from build123d import *

# Parameters (mm, degrees)
SKETCH1_R           = 18
BOSS_EXTRUDE1_DEPTH = 70
SKETCH2_R           = 2.5
BOSS_EXTRUDE2_DEPTH = 16
SKETCH3_R           = 9.5
SKETCH3_R_2         = 2.5
BOSS_EXTRUDE3_DEPTH = 25
SKETCH4_R           = 9.5
SKETCH4_R_2         = 4
BOSS_EXTRUDE4_DEPTH = 10


with BuildPart() as part:
    # Sketch1 → Boss-Extrude1 (new body)
    with BuildSketch(Plane.XY):
        Circle(SKETCH1_R)
    extrude(amount=BOSS_EXTRUDE1_DEPTH)

    # Sketch2 → Boss-Extrude2 (add)
    with BuildSketch(Plane.XY.offset(70)):
        Circle(SKETCH2_R)
    extrude(amount=BOSS_EXTRUDE2_DEPTH)

    # Sketch3 → Boss-Extrude3 (add)
    with BuildSketch(Plane.XY.offset(70)):
        Circle(SKETCH3_R)
        Circle(SKETCH3_R_2, mode=Mode.SUBTRACT)
    extrude(amount=BOSS_EXTRUDE3_DEPTH)

    # Sketch4 → Boss-Extrude4 (add)
    with BuildSketch(Plane.XY.offset(95)):
        Circle(SKETCH4_R)
        Circle(SKETCH4_R_2, mode=Mode.SUBTRACT)
    extrude(amount=BOSS_EXTRUDE4_DEPTH)


solid = part.part
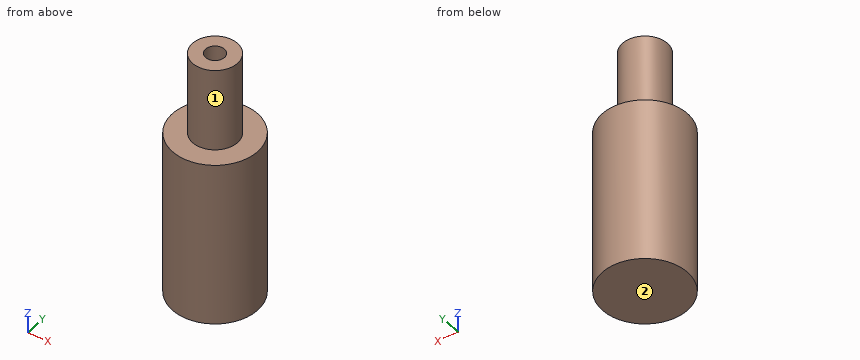
The listing builds one solid part. Answer for the finished solid, in the listing's coordinates (mm). Face numbers are marked on the shaded views. A direction names the side the tool comes from. Coordinates: 2 decimals unless noted, no trailing zeros. Order: outer loops, then holes, each group sorted by start corner. A loop starts at its lowest first (then second) coordinate and runs counter-clockwise, first axis right, second up.
Q1. Which of the six approach directions +Z, -Z, +X, -X, +Y, -Y give full straight-line access (tool end or side, diameter ignored) to the marked faces 1 and 2?
Q2. Given P1, Ø1, axis at y = -11, z = 27, coming from the -X side; P2, Ø2.5, axis at x = 1, y = 1, coming from the +Z side; P3, Ø1, axis at x = -10.5, y = -1.5, coming from the -Z side; P4, Ø6, axis at x = -13, z = 50, coming from the -Y side, each flat-ended and moving along its own axis, determine where each tip first touches the part or whether it passes through.
Q3. A cutting plane is placed at D-D, the plane z = 61. Write down the section's boundary in (x, y).
Q4. A cutting plane is placed at B-B, the plane z = 88.5. Write down the section's boundary in (x, y), and give its area (3 significant figures).
Q5. Consider line 1 (Y direction, x = 0, z = 89.5); line 2 (Y direction, x = 0, z = 101.5); line 3 (Z direction, x = 11, y = 11.5). Determine where each line is inside the solid, lowest interval first.
Q6. A cutting plane is placed at A-A, the plane x = 0. Write down the section's boundary in (y, z), and give its area (3 significant figures).
Answers follow:
1. face 1: +Z
1. face 2: -Z, +X, -X, +Y, -Y
2. P1: stops at x = -14.62
2. P2: stops at z = 95
2. P3: stops at z = 0
2. P4: stops at y = -14.97
3. outline: circle Ø36 at (0, 0)
4. outline: circle Ø19 at (0, 0); hole circle Ø5 at (0, 0)
4. area: 264 mm2
5. line 1: y = -9.5 to -2.5, 2.5 to 9.5
5. line 2: y = -9.5 to -4, 4 to 9.5
5. line 3: z = 0 to 70
6. outline: (-18, 0) - (18, 0) - (18, 70) - (9.5, 70) - (9.5, 105) - (4, 105) - (4, 95) - (2.5, 95) - (2.5, 86) - (-2.5, 86) - (-2.5, 95) - (-4, 95) - (-4, 105) - (-9.5, 105) - (-9.5, 70) - (-18, 70) - close
6. area: 3,060 mm2
